Verification items for the finished model (mm, model axes). Face numbers are marked on the shaded views. A direction names the side the tool comes from. Coordinates: 2 decimals unless noted, no trailing zeros. Order: outer loops, then holes, each group sorted by start corner. A loop starts at its lowest first (then second) coordinate and runs counter-clockwise, first axis right, second up.
Q1. Thickness scan on line 1 (Z direction, x = 0.5, y = 2.75); line 2 (Y direction, x = -2.5, z = 1.75); line 3 (Y direction, x = -1.5, z = 9). Record the ranges inside material, lowest first.
Q2. Depth check by flat-ended pin: P1, Ø1.5, axis at y = -0.5, z = 15, coming from the +X side. Enter the tip coordinate at first touch or a pass-through.
Q3. Cross-section at D-D, the plane z = 9. Record the boundary of the cut face in (x, y), and give its area (3 significant figures).
Q4. Set-up check for the marked faces 1, 2 and 3: record each of +Z, -Z, +X, -X, +Y, -Y from which the full face is reachable in a straight line by a thin tool's end or side.
Q5. Cross-section at C-C, the plane z = 18.25. Record the boundary of the cut face in (x, y), and give its area (3 significant figures).
Q6. Cross-section at B-B, the plane y = 0. Record the boundary of the cut face in (x, z), and give its area (3 significant figures).
Q7. Cross-section at A-A, the plane x = 0. Record the boundary of the cut face in (y, z), and give its area (4 significant figures).
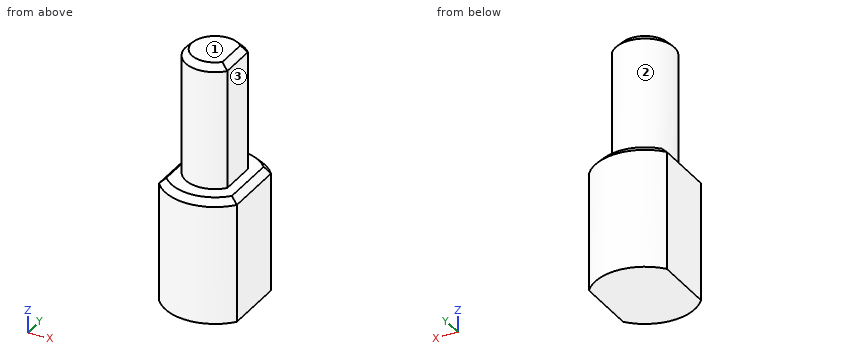
Autodesk Inventor part; units mm, degrees
ref_plane "YZ Plane" through (0, 0, 0) normal (1, 0, 0) x (0, 1, 0)
ref_plane "XZ Plane" through (0, 0, 0) normal (0, 1, 0) x (-1, 0, 0)
ref_plane "XY Plane" through (0, 0, 0) normal (0, 0, 1) x (1, 0, 0)
sketch "Sketch1" plane through (0, 0, 0) normal (0, 0, 1) x (1, 0, 0)
  circle A0 centre (0, 0) radius 4
  line L0 (3.1225, 2.5) -> (3.1225, -2.5)
  line L1 (-3.1225, 2.5) -> (-3.1225, -2.5)
  dimension "d0" = 8
  dimension "d1" = 5
  dimension "d2" = 5
extrude "Extrusion1" add sketch "Sketch1" along normal blind 10 contours L0 A0 L1
sketch "Sketch2" plane through (0, 0, 10) normal (0, 0, 1) x (1, 0, 0)
  circle A0 centre (0, 0) radius 2.35
  line L0 (1.809, 1.5) -> (1.809, -1.5)
  dimension "d5" = 4.7
  dimension "d6" = 3
extrude "Extrusion2" add sketch "Sketch2" along normal blind 10 contours L0 A0 picked at (0.4227, 0)
chamfer "Chamfer1" distance 0.5 angle 45 6 edges at (1.809, 0, 20) (-2.35, 0, 20) (3.1225, 0, 10) (0, 4, 10) (0, -4, 10) (-3.1225, 0, 10)
properties part number "Shaft_Peg"
Check values:
1. line 1: z = 0 to 10
1. line 2: y = -3.12 to 3.12
1. line 3: y = -3.71 to 3.71
2. P1: stops at x = 1.81
3. outline: (-3.12, -2.5) arc R4 ccw to (3.12, -2.5) - (3.12, 2.5) arc R4 ccw to (-3.12, 2.5) - close
3. area: 44.3 mm2
4. face 1: +Z, +X, -X, +Y, -Y
4. face 2: +Z
4. face 3: +Z, +X, +Y, -Y
5. outline: (1.81, -1.5) - (1.81, 1.5) arc R2.35 ccw (long way) to start
5. area: 16.2 mm2
6. outline: (-3.12, 0) - (3.12, 0) - (3.12, 9.5) - (2.62, 10) - (1.81, 10) - (1.81, 19.5) - (1.31, 20) - (-1.85, 20) - (-2.35, 19.5) - (-2.35, 10) - (-2.62, 10) - (-3.12, 9.5) - close
6. area: 104 mm2
7. outline: (-4, 0) - (4, 0) - (4, 9.5) - (3.5, 10) - (2.35, 10) - (2.35, 19.5) - (1.85, 20) - (-1.85, 20) - (-2.35, 19.5) - (-2.35, 10) - (-3.5, 10) - (-4, 9.5) - close
7. area: 126.5 mm2
